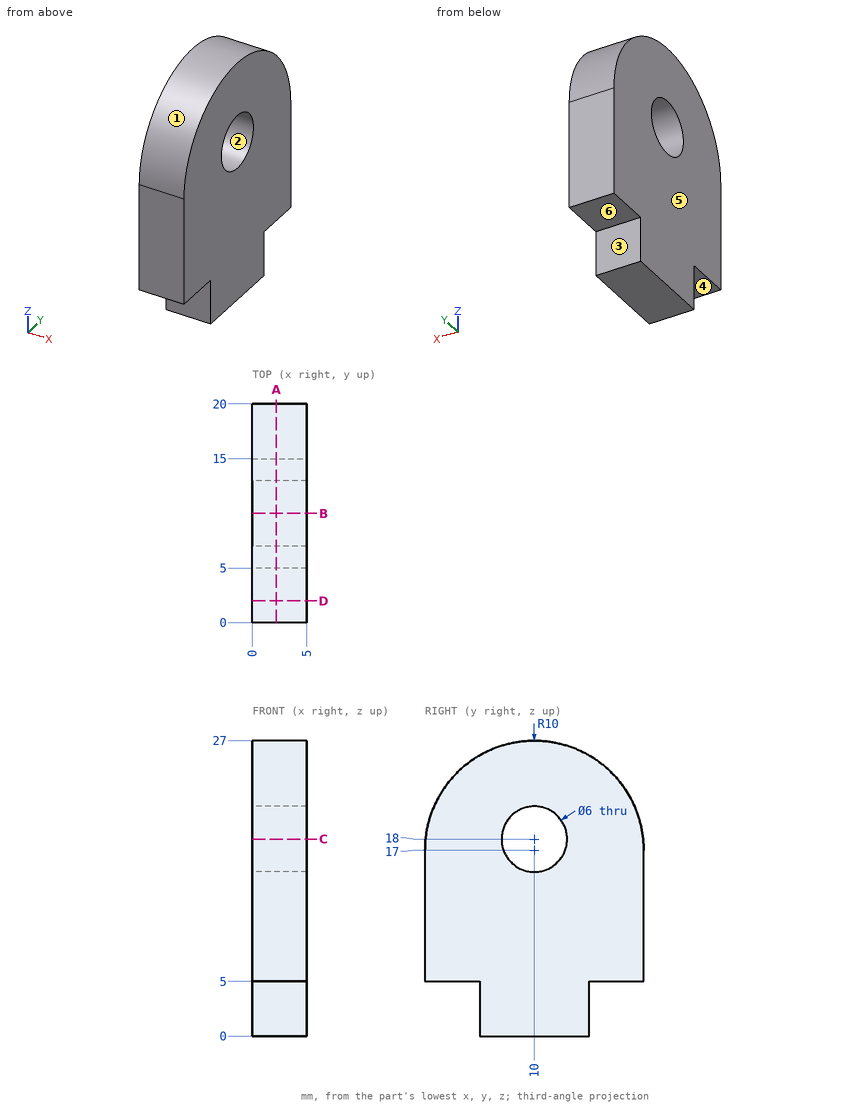
Check sheet for the drawn part. Datum: minimum x, y, z corner. Units: mm. A direction names the side the tool comes from. Give positions to 0.01 mm unless a question says otherwise; leave off trailing zeros. Loops run counter-clockwise (first coordinate to the right, second up) from the corner with the lowest first, then second, coordinate; pieces in that order, holes last. Notation, with made-up numbers: M 1,63.25 L 33,63.25 A13 ccw 33,80.25 Z; hole C -23,-8.5 d7. An arc over 180 degrees is marked long. Answer as CSV lines item,"result".
Item 1: Sectioned sample at D-D, the plane y = 2. Enter the section's corners in (x, z).
Reply:
outline,"M 0,5 L 5,5 L 5,23 L 0,23 Z"
Item 2: Depth check by flat-ended pin: pin 1 Ø1 at (x, y) = (4.5, 5) entering from +Z; pin 2 Ø2.5 at (x, y) = (2, 1.5) entering from -Z; pin 3 Ø2.5 at (x, z) = (1.5, 3.5) entering from +Y. Enter the tip coordinate at first touch or a pass-through.
Reply:
pin 1,"z = 25.93"
pin 2,"z = 5"
pin 3,"y = 15"
Item 3: Draft check along Z on the marked faces 1, 2 and 3. Enter one of: pulls with the +Z half, pulls with the -Z half, needs draft (parallel to the pull), parting line crosses it, or undercut.
Reply:
face 1,"pulls with the +Z half"
face 2,"undercut"
face 3,"needs draft"
Item 4: Sectioned sample at C-C, the plane z = 18. Enter the section's corners in (x, y).
Reply:
outline,"M 0,0.05 L 5,0.05 L 5,7 L 0,7 Z; M 0,13 L 5,13 L 5,19.95 L 0,19.95 Z"
Item 5: Scan lines: L1, parallel to Y at x = 2, z = 18; L2, parallel to Z at x = 0.75, y = 10.5; L3, parallel to Y at x = 0.3, z = 1. Record each from-to range of solid material in increasing order.
Reply:
L1,"0.05 to 7, 13 to 19.95"
L2,"0 to 15.04, 20.96 to 26.99"
L3,"5 to 15"
Item 6: Set-up check for the marked faces 4, 5 and 6: record each of +Z, -Z, +X, -X, +Y, -Y from which the full face is reachable in a straight line by a thin tool's end or side.
Reply:
face 4,"-Z, +X, -X, -Y"
face 5,"+Z, -Z, -X, +Y, -Y"
face 6,"-Z, +X, -X, +Y"
Item 7: Sectioned sample at A-A, the plane x = 2.2. Enter the section's corners in (y, z), then the cut area to 3 significant figures.
Reply:
outline,"M 0,5 L 5,5 L 5,0 L 15,0 L 15,5 L 20,5 L 20,17 A10 ccw 0,17 Z; hole C 10,18 d6"
area,"419 mm^2"
Item 8: Sectioned sample at B-B, the plane y = 10. Enter the section's corners in (x, z), then the cut area to 3 significant figures.
Reply:
outline,"M 0,0 L 5,0 L 5,15 L 0,15 Z; M 0,21 L 5,21 L 5,27 L 0,27 Z"
area,"105 mm^2"
